For this review, take the finished solid that the model builds, in its own axes (mm). Round coordinates to 2 decimals unless told otherwise and drop trailing zeros. Write each loop counter-clockwise with the first axis right and the second up, starting at its lowest first coordinate (ties: lowest second). Pieces come first, ordered by that corner, then holes. Notation, with made-up numbers: (79.25, 62.5) -> (87.25, 62.5) arc R35 cw to (87.25, 99.5) -> close; hole circle Ø8 at (57.25, 31.25). An arc over 180 degrees is marked (long way). Answer in a Markdown table with one row per item.
from build123d import *

# Parameters (mm, degrees)
F0_R     = 30.226
F1_DEPTH = 19.05
F3_D     = 5.0038
F3_DEPTH = 14.224
F3_TIP   = 1.5032931827


with BuildPart() as f1:
    # F0 (on Right) → F1 (new body)
    with BuildSketch(Plane.YZ):
        with BuildLine():
            Line((304.8, -482.6), (304.8, 622.3))
            Line((304.8, 622.3), (124.6301678728, 622.3))
            ThreePointArc((124.6301678728, 622.3), (114.5071784324, 621.2811719909), (104.7902356525, 618.2655545193))
            Line((104.7902356525, 618.2655545193), (-304.8, 444.5))
            Line((-304.8, 444.5), (-304.8, 396.875))
            Line((-304.8, 396.875), (-304.8, -622.3))
            Line((-304.8, -622.3), (304.8, -622.3))
            Line((304.8, -622.3), (304.8, -482.6))
        make_face()
        with Locations((203.2, -482.6)):
            Circle(F0_R, mode=Mode.SUBTRACT)
    extrude(amount=F1_DEPTH)

    # F3
    with Locations(Plane.YZ.offset(19.05)):
        with Locations((-203.2, 136.525), (-203.2, 104.775), (-203.2, 73.025), (-203.2, 41.275), (-203.2, 9.525), (-203.2, -22.225), (-203.2, -53.975), (-203.2, -85.725), (-203.2, -117.475), (-203.2, -149.225), (-203.2, -180.975), (-203.2, -212.725), (-203.2, -244.475), (-203.2, -276.225), (-203.2, -307.975), (-203.2, -339.725), (-203.2, -371.475), (-203.2, -403.225), (203.2, -403.225), (203.2, -371.475), (203.2, -339.725), (203.2, -307.975), (203.2, -276.225), (203.2, -244.475), (203.2, -212.725), (203.2, -180.975), (203.2, -149.225), (203.2, -117.475), (203.2, -85.725), (203.2, -53.975), (203.2, -22.225), (203.2, 9.525), (203.2, 41.275), (203.2, 73.025), (203.2, 104.775), (203.2, 136.525)):
            Hole(F3_D / 2, depth=F3_DEPTH)
            with Locations((0, 0, -(F3_DEPTH + F3_TIP / 2))):  # 118° drill point
                Cone(0, F3_D / 2, F3_TIP, mode=Mode.SUBTRACT)


solid = f1.part
1) Clearance check with flat-ended pins moving along their axes: pin 1 Ø4.5 at (y, z) = (203.2, -403.225) entering from +X; pin 2 Ø3 at (x, y) = (16, -4.5) entering from +Z; pin 3 Ø10 at (x, y) = (10, -116.5) entering from +Z. State where each tip first meets the part, or that it passes through.
Solved:
| item | result |
|---|---|
| pin 1 | x = 4.67 |
| pin 2 | z = 572.54 |
| pin 3 | z = 526.51 |
2) Consider section C-C on y = -3. State the section outline as (x, z) points, then the cut area to 3 significant figures.
Solved:
| item | result |
|---|---|
| outline | (0, -622.3) -> (19.05, -622.3) -> (19.05, 572.54) -> (0, 572.54) -> close |
| area | 22,800 mm² |
3) Consider section B-B on y = -70.5. State the section outline as (x, z) points, then the cut area to 3 significant figures.
Solved:
| item | result |
|---|---|
| outline | (0, -622.3) -> (19.05, -622.3) -> (19.05, 543.9) -> (0, 543.9) -> close |
| area | 22,200 mm² |
4) Mouldability with a two-part tool opening along Y and no side actions: class faces 1 (the flat face through (0, -4, 9)), 2 (the flat face through (9.39, -97.14, 532.6)), 3 (the cylindrical face through (9.39, 199.27, -452.63)) as pulls with the +Y half, pulls with the -Y half, needs draft (parallel to the pull), parting line crosses it, or undercut.
Solved:
| item | result |
|---|---|
| face 1 | needs draft |
| face 2 | pulls with the -Y half |
| face 3 | undercut |
5) For line 1 (Y direction, x = 8, z = -371.5); line 2 (Y direction, x = 6.25, z = -497); line 3 (Z direction, x = 3.5, y = -213), list the stretches that pass through material, from the lowest coordinate up. Write a range as [from, to].
Solved:
| item | result |
|---|---|
| line 1 | [-304.8, -205.7], [-200.7, 200.7], [205.7, 304.8] |
| line 2 | [-304.8, 176.62], [229.78, 304.8] |
| line 3 | [-622.3, 483.45] |
6) Consider section A-A on z = -482.6. State the section outline as (x, y) points, then the cut area to 3 significant figures.
Solved:
| item | result |
|---|---|
| outline | (0, -304.8) -> (19.05, -304.8) -> (19.05, 172.97) -> (0, 172.97) -> close; (0, 233.43) -> (19.05, 233.43) -> (19.05, 304.8) -> (0, 304.8) -> close |
| area | 10,500 mm² |
